```python
from build123d import *

# Parameters (mm, degrees)
SKETCH1_R           = 3.048
BOSS_EXTRUDE1_DEPTH = 5.3975
BOSS_EXTRUDE1_DRAFT = -10
SKETCH3_R           = 3.048
BOSS_EXTRUDE2_DEPTH = 14.986
SKETCH4_R           = 3.048
BOSS_EXTRUDE3_DEPTH = 1.5875
BOSS_EXTRUDE3_DRAFT = -75
BOSS_EXTRUDE5_DEPTH = 3.175


with BuildPart() as part:
    # Sketch1 → Boss-Extrude1 (with draft: the straight prism first)
    with BuildSketch(Plane(origin=(0, 0, 0), x_dir=(1, 0, 0), z_dir=(0, 1, 0))):
        Circle(SKETCH1_R)
    extrude(amount=-BOSS_EXTRUDE1_DEPTH)
    # Boss-Extrude1: the draft: its side faces are tilted about the plane it starts from
    boss_extrude1_sides = [part.faces().sort_by_distance(p)[0] for p in [
        (-3.048, -2.69875, 0),
    ]]
    draft(boss_extrude1_sides, Plane(origin=(0, 0, 0), x_dir=(1, 0, 0), z_dir=(0, 1, 0)), BOSS_EXTRUDE1_DRAFT)

    # Sketch3 → Boss-Extrude2 (add)
    with BuildSketch(Plane(origin=(0, 0, 0), x_dir=(1, 0, 0), z_dir=(0, 1, 0))):
        with Locations(Location((0, 0, 0), (0, 0, 270))):
            Circle(SKETCH3_R)
    extrude(amount=BOSS_EXTRUDE2_DEPTH)


with BuildPart() as boss_extrude3_tool:
    # Sketch4 → Boss-Extrude3 (with draft: the straight prism first)
    with BuildSketch(Plane(origin=(0, 14.986, 0), x_dir=(1, 0, 0), z_dir=(0, 1, 0))):
        with Locations(Location((0, 0, 0), (0, 0, 270))):
            Circle(SKETCH4_R)
    extrude(amount=BOSS_EXTRUDE3_DEPTH)
    # Boss-Extrude3: the draft: its side faces are tilted about the plane it starts from
    boss_extrude3_sides = [boss_extrude3_tool.faces().sort_by_distance(p)[0] for p in [
        (0, 15.77975, -3.048),
    ]]
    draft(boss_extrude3_sides, Plane(origin=(0, 14.986, 0), x_dir=(1, 0, 0), z_dir=(0, 1, 0)), BOSS_EXTRUDE3_DRAFT)


with BuildPart() as part_1:
    add(part.part)

    # Boss-Extrude3: add boss_extrude3_tool
    add(boss_extrude3_tool.part)

    # Sketch6 → Boss-Extrude5 (add)
    with BuildSketch(Plane(origin=(0, 16.5735, 0), x_dir=(1, 0, 0), z_dir=(0, 1, 0))):
        Polygon((3.317975387, 8.928418916), (0.66814778, 9.501536904), (-2.035809185, 9.304896881), (-4.574836998, 8.35442945), (-6.743238725, 6.727135831), (-8.365343354, 4.554849675), (-9.309737615, 2.013556687), (-9.499912302, -0.690862688), (-8.920460592, -3.339312478), (-7.618326217, -5.71723103), (-5.69900036, -7.631973526), (-3.317975387, -8.928418916), (-0.66814778, -9.501536904), (2.035809185, -9.304896881), (4.574836998, -8.35442945), (6.743238725, -6.727135831), (8.365343354, -4.554849675), (9.309737615, -2.013556687), (9.499912302, 0.690862688), (8.920460592, 3.339312478), (7.618326217, 5.71723103), (5.69900036, 7.631973526), align=None)
    extrude(amount=BOSS_EXTRUDE5_DEPTH)


solid = part_1.part
```
The listing builds one solid part. Answer for the finished solid, in the listing's coordinates (mm). A direction names the side the tool comes from. Round coordinates to 2 decimals unless told otherwise and drop trailing zeros. Loops run counter-clockwise (first coordinate to the right, second up) from the corner with the lowest first, then second, coordinate; pieces in that order, holes last.
Q1. Section A-A, the plane z = 0 is taken. Determine the outline of the cut face in (x, y).
Q2. Which of the six approach directions +Z, -Z, +X, -X, +Y, -Y give full straight-line access (tool end or side, diameter ignored) to faces 1 (the face through (7.7, 16.574, 4.9)), 2 (the face through (-3.288, 18.139, -8.836))?
Q3. Section B-B, the plane x = 0 is taken. Determine the outline of the cut face in (y, z), then the cut area to 3 significant figures.
Q4. Section D-D, the plane y = -2.25 is taken. Determine the outline of the cut face in (x, z).
Q5. Section C-C, the plane y = 6.5 is taken. Determine the outline of the cut face in (x, z), then the cut area to 3 significant figures.
Q6. Given pin 1 Ø10 at (y, z) = (2, 6.5) entering from +X; pin 2 Ø5 at (y, z) = (17, -5) entering from +X; pin 3 Ø3 at (y, z) = (7.5, -1.5) entering from -X, each flat-ended and moving along its own axis, determine where each tip first touches the part or whether it passes through.
Q7. Find the intervals of material crossed by line 1 (Y direction, x = -7, z = 6); line 2 (Z direction, x = 0, y = 5); line 3 (X direction, y = 2.5, z = 1), in increasing order.
Completed:
1. outline: (-9.45, 16.57) - (-8.97, 16.57) - (-3.05, 14.99) - (-3.05, 0) - (-2.1, -5.4) - (2.1, -5.4) - (3.05, 0) - (3.05, 14.99) - (8.97, 16.57) - (9.45, 16.57) - (9.45, 19.75) - (-9.45, 19.75) - close
2. face 1: -Y
2. face 2: -Z, -X, +Y, -Y
3. outline: (-5.4, -2.1) - (0, -3.05) - (14.99, -3.05) - (16.57, -8.97) - (16.57, -9.45) - (19.75, -9.45) - (19.75, 9.45) - (16.57, 9.45) - (16.57, 8.97) - (14.99, 3.05) - (0, 3.05) - (-5.4, 2.1) - close
3. area: 198 mm2
4. outline: circle Ø5.3 at (0, 0)
5. outline: circle Ø6.1 at (0, 0)
5. area: 29.2 mm2
6. pin 1: stops at x = 2.65
6. pin 2: stops at x = 9.1
6. pin 3: stops at x = -3.05
7. line 1: y = 16.57 to 19.75
7. line 2: z = -3.05 to 3.05
7. line 3: x = -2.88 to 2.88
